```python
from build123d import *

# Parameters (mm, degrees)
SKETCH3_R           = 4
SKETCH3_R_2         = 15
BOSS_EXTRUDE1_DEPTH = 8


with BuildPart() as part:
    # Sketch3 → Boss-Extrude1 (new body)
    with BuildSketch(Plane(origin=(0, 0, 0), x_dir=(1, 0, 0), z_dir=(0, 1, 0))):
        with BuildLine():
            Line((-85.097948738, 70.953076893), (12.255128155, 27.382692233))
            ThreePointArc((12.255128155, 27.382692233), (30, 0), (12.255128155, -27.382692233))
            Line((12.255128155, -27.382692233), (-85.097948738, -70.953076893))
            ThreePointArc((-85.097948738, -70.953076893), (-101.735350926, -62.506299791), (-90, -48))
            ThreePointArc((-90, -48), (-50, 0), (-90, 48))
            ThreePointArc((-90, 48), (-101.735350926, 62.506299791), (-85.097948738, 70.953076893))
        make_face()
        with Locations(Location((-90, 60, 0), (0, 0, 270))):
            Circle(SKETCH3_R, mode=Mode.SUBTRACT)
        with Locations(Location((-90, -60, 0), (0, 0, 270))):
            Circle(SKETCH3_R, mode=Mode.SUBTRACT)
        with Locations(Location((22.5, 0, 0), (0, 0, 270))):
            Circle(SKETCH3_R, mode=Mode.SUBTRACT)
        with Locations(Location((-22.5, 0, 0), (0, 0, 270))):
            Circle(SKETCH3_R, mode=Mode.SUBTRACT)
        with Locations(Location((0, 0, 0), (0, 0, 270))):
            Circle(SKETCH3_R_2, mode=Mode.SUBTRACT)
    extrude(amount=BOSS_EXTRUDE1_DEPTH)


solid = part.part
```
Geometry: final body of the model. Coordinates: model frame, mm. Give positions to 0.01 mm unless a question says otherwise; leave off trailing zeros. Write each loop counter-clockwise with the first axis right and the second up, starting at its lowest first coordinate (ties: lowest second). Pieces come first, ordered by that corner, then holes.
1. Section query B-B, the plane x = -22.5. Return loops of the section in (y, z).
2. Section query C-C, the plane z = 60. Return loops of the section in (x, y).
3. Section query D-D, the plane z = 25. Return loops of the section in (x, y).
4. Pin query (flat end, axial travel): P1, Ø10.5, axis at x = -90, z = -60, coming from the -Y side; P2, Ø4, axis at y = 4, z = 23.5, coming from the -X side; P3, Ø1, axis at x = -2.5, y = 4.5, coming from the +Z side; P4, Ø6.5, axis at x = -22.5, z = 0, coming from the +Y side. Return the tip coordinate at first contact, or that it passes through.
5. Draft query along Z for faces 1 (the flat face through (-37.1, 3.94, -49.47)), 2 (the flat face through (-35, 0, -1)), 3 (the cylindrical face through (-101.794, 3.944, -62.213)). Return one class per face: released by +Z, released by -Z, zero draft, split by the parting line, or undercut.
6. Line query: probe 1 along X at (y, z) = (4.5, 0); probe 2 along Z at (x, y) = (-89, 5.5); probe 3 along X at (y, z) = (4.5, -61.5). Output: solid intervals per line, ascending.
7. Section query A-A, the plane z = 0. Return loops of the section in (x, y), then the cut area to 3 significant figures.
Computed:
1. outline: (0, -42.94) - (8, -42.94) - (8, -4) - (0, -4) - close; (0, 4) - (8, 4) - (8, 42.94) - (0, 42.94) - close
2. outline: (-102, 0) - (-94, 0) - (-94, 8) - (-102, 8) - close; (-86, 0) - (-60.62, 0) - (-60.62, 8) - (-86, 8) - close
3. outline: (-56.89, 0) - (16.58, 0) - (16.58, 8) - (-56.89, 8) - close
4. P1: stops at y = 0
4. P2: stops at x = -57.19
4. P3: stops at z = 34.21
4. P4: passes through
5. face 1: released by -Z
5. face 2: zero draft
5. face 3: undercut
6. probe 1: x = -50 to -26.5, -18.5 to -15, 15 to 18.5, 26.5 to 30
6. probe 2: z = -71.96 to -63.87, -56.13 to -47.81, 47.81 to 56.13, 63.87 to 71.96
6. probe 3: x = -101.91 to -93.71, -86.29 to -63.98
7. outline: (-50, 0) - (-26.5, 0) - (-26.5, 8) - (-50, 8) - close; (-18.5, 0) - (-15, 0) - (-15, 8) - (-18.5, 8) - close; (15, 0) - (18.5, 0) - (18.5, 8) - (15, 8) - close; (26.5, 0) - (30, 0) - (30, 8) - (26.5, 8) - close
7. area: 272 mm2
